Autodesk Inventor part; units mm, degrees
ref_plane "YZ Plane" through (0, 0, 0) normal (1, 0, 0) x (0, 1, 0)
ref_plane "XZ Plane" through (0, 0, 0) normal (0, 1, 0) x (-1, 0, 0)
ref_plane "XY Plane" through (0, 0, 0) normal (0, 0, 1) x (1, 0, 0)
sketch "Szkic1" plane through (0, 0, 0) normal (0, 0, 1) x (1, 0, 0)
  line L0 (-9.6574, 2.8417) -> (18.3426, 2.8417)
  line L1 (18.3426, 2.8417) -> (18.3426, -6.1583)
  line L2 (18.3426, -6.1583) -> (-9.6574, -6.1583)
  line L3 (-9.6574, -6.1583) -> (-9.6574, 2.8417)
  line L4 (-1.1574, -6.1583) -> (-1.1574, -7.6583)
  line L5 (-1.1574, -7.6583) -> (9.8426, -7.6583)
  line L6 (9.8426, -7.6583) -> (9.8426, -6.1583)
  point P0 (0, 0)
  point P1 (4.3426, -2.4083)
  dimension "d0" = 28
  dimension "d1" = 9
  dimension "d2" = 1.5
  dimension "d3" = 11
  dimension "d4" = 8.5
  dimension "d20" = 14
  dimension "d21" = 10.5
  dimension "d22" = 5.25
extrude "Wyciągnięcie proste1" add sketch "Szkic1" along normal blind 4.75
sketch "Szkic2" plane through (0, 0, 4.75) normal (0, 0, 1) x (1, 0, 0)
  line L0 (-9.6574, -6.1583) -> (-1.1574, -6.1583)
  line L1 (9.8426, -6.1583) -> (18.3426, -6.1583)
  line L2 (18.3426, 2.8417) -> (-9.6574, 2.8417)
  line L3 (-9.6574, 2.8417) -> (-9.6574, -6.1583)
  line L4 (18.3426, -6.1583) -> (18.3426, 2.8417)
  line L5 (14.0926, -3.1583) -> (14.0926, -0.1583) construction
  line L6 (15.7426, -3.1583) -> (15.7426, -0.1583)
  line L7 (12.4426, -0.1583) -> (12.4426, -3.1583)
  arc A0 (12.4426, -3.1583) -> (15.7426, -3.1583) centre (14.0926, -3.1583) ccw
  arc A1 (15.7426, -0.1583) -> (12.4426, -0.1583) centre (14.0926, -0.1583) ccw
  line L8 (-5.4074, -3.1583) -> (-5.4074, -0.1583) construction
  line L9 (-3.7574, -3.1583) -> (-3.7574, -0.1583)
  line L10 (-7.0574, -0.1583) -> (-7.0574, -3.1583)
  arc A2 (-7.0574, -3.1583) -> (-3.7574, -3.1583) centre (-5.4074, -3.1583) ccw
  arc A3 (-3.7574, -0.1583) -> (-7.0574, -0.1583) centre (-5.4074, -0.1583) ccw
  point P0 (0, 0)
  point P1 (-5.4074, -1.6583)
  point P2 (14.0926, -1.6583)
  dimension "d7" = 4.5
  dimension "d8" = 4.5
  dimension "d9" = 9
  dimension "d10" = 8.5
  dimension "d11" = 4.25
  dimension "d12" = 4.25
  dimension "d13" = 1.5
  dimension "d14" = 3.3
  dimension "d15" = 1.5
  dimension "d16" = 3.3
extrude "Wyciągnięcie proste2" cut sketch "Szkic2" against normal blind 10
fillet "Zaokrąglenie1" radius 2.5 4 edges at (-9.6574, 2.8417, 2.375) (-9.6574, -6.1583, 2.375) (18.3426, -6.1583, 2.375) (18.3426, 2.8417, 2.375)
hole "Otwór1" at (4.3426, -2.4083, 0) direction (0, 0, 1) diameter 3.25 end through all
equation "\"d4\" = -0.5 * d3 + 0.5 * d0"
properties part number "3DP_ABS_Extruder_Tensioning_Arm_Screw_Mount"
Source: CAD feature listing. Evaluate the final solid. Frame: model axes, mm. A direction names the side the tool comes from. Round coordinates to 2 decimals unless told otherwise and drop trailing zeros. Order: outer loops, then holes, each group sorted by start corner. A loop starts at its lowest first (then second) coordinate and runs counter-clockwise, first axis right, second up. Notation, with made-up numbers: (-31.5, 22.5) -> (2.5, 22.5) arc R25 cw to (2.5, 38.5) -> close; hole circle Ø9 at (57.5, 73.5). An arc over 180 degrees is marked (long way). One line per item, written item: value. Start each with the question number.
Q1. Access query for faces 1 (the flat face through (-1.157, -7, 2)), 2 (the flat face through (18.343, -2, 2)), 3 (the cylindrical face through (14.056, -4.808, 2.408)), 4 (the flat face through (13, -6.158, 2)). Directions: +Z, -Z, +X, -X, +Y, -Y. A direction counts if a zero-diameter tool reaches every point of the face in a straight line with its end or side. Return the directions, or none.
Q2. Section query B-B (x = 3.5). Return the cut outline in (y, z).
Q3. Material intervals for probe 1 along X at (y, z) = (-0.75, 3); probe 2 along X at (y, z) = (-2.5, 2.05); probe 3 along X at (y, z) = (-3.5, 1.8), sorted ascending.
Q4. Section query D-D (x = 14.75). Return the cut outline in (y, z).
Q5. Draft query along Y for faces 5 (the flat face through (-4, -6.158, 2)), 6 (the flat face through (4, 0, 0)), 7 (the cylindrical face through (-5.37, 1.49, 2.41)). Return one class per face: pulls with the +Y half, pulls with the -Y half, needs draft (parallel to the pull), parting line crosses it, or undercut.
Q6. Pin query (flat end, axial travel): pin 1 (2.5 mm diameter, centred on x = 14, z = 3, fed in from -Y); pin 2 (1.2 mm diameter, centred on y = -7, z = 3.5, fed in from +X). Return the tip coordinate at first contact, or that it passes through.
Q7. Section query C-C (z = 3.35). Return the cut outline in (x, y) (3 decimals).
Q8. Section query A-A (y = -0.5). Return the cut outline in (x, z), plus the area to 3 significant figures.
Findings below:
1. face 1: +Z, -Z, -X, -Y
1. face 2: +Z, -Z, +X, +Y, -Y
1. face 3: +Z, -Z
1. face 4: +Z, -Z, +X, -Y
2. outline: (-7.66, 0) -> (-3.8, 0) -> (-3.8, 4.75) -> (-7.66, 4.75) -> close; (-1.02, 0) -> (2.84, 0) -> (2.84, 4.75) -> (-1.02, 4.75) -> close
3. probe 1: -9.66 to -7.06, -3.76 to 12.44, 15.74 to 18.34
3. probe 2: -9.66 to -7.06, -3.76 to 2.72, 5.97 to 12.44, 15.74 to 18.34
3. probe 3: -9.66 to -7.02, -3.79 to 3.14, 5.55 to 12.48, 15.71 to 18.34
4. outline: (-6.16, 0) -> (-4.67, 0) -> (-4.67, 4.75) -> (-6.16, 4.75) -> close; (1.36, 0) -> (2.84, 0) -> (2.84, 4.75) -> (1.36, 4.75) -> close
5. face 5: pulls with the -Y half
5. face 6: needs draft
5. face 7: undercut
6. pin 1: y = -6.16
6. pin 2: x = 9.84
7. outline: (-9.657, -3.658) arc R2.5 ccw to (-7.157, -6.158) -> (-1.157, -6.158) -> (-1.157, -7.658) -> (9.843, -7.658) -> (9.843, -6.158) -> (15.843, -6.158) arc R2.5 ccw to (18.343, -3.658) -> (18.343, 0.342) arc R2.5 ccw to (15.843, 2.842) -> (-7.157, 2.842) arc R2.5 ccw to (-9.657, 0.342) -> close; hole (-7.057, -3.158) arc R1.65 ccw to (-3.757, -3.158) -> (-3.757, -0.158) arc R1.65 ccw to (-7.057, -0.158) -> close; hole circle Ø3.25 at (4.343, -2.408); hole (12.443, -3.158) arc R1.65 ccw to (15.743, -3.158) -> (15.743, -0.158) arc R1.65 ccw to (12.443, -0.158) -> close
8. outline: (-9.66, 0) -> (-7.06, 0) -> (-7.06, 4.75) -> (-9.66, 4.75) -> close; (-3.76, 0) -> (12.44, 0) -> (12.44, 4.75) -> (-3.76, 4.75) -> close; (15.74, 0) -> (18.34, 0) -> (18.34, 4.75) -> (15.74, 4.75) -> close
8. area: 102 mm²
